```python
from build123d import *

# Parameters (mm, degrees)
SKETCH1_W             = 101.6
SKETCH1_H             = 25.4
BOSS_EXTRUDE1_DEPTH   = 9.525
SKETCH2_W             = 9.525
SKETCH2_H             = 3.175
SKETCH2_W_2           = 42.8625
SKETCH2_H_2           = 4.7625
CUT_EXTRUDE1_DEPTH    = 106.159144277
F_8_32_TAPPED_HOLE1_D = 3.4544


with BuildPart() as part:
    # Sketch1 → Boss-Extrude1 (new body)
    with BuildSketch(Plane.XY):
        with Locations((50.8, 12.7)):
            Rectangle(SKETCH1_W, SKETCH1_H)
    extrude(amount=BOSS_EXTRUDE1_DEPTH)

    # Sketch2 → Cut-Extrude1 (cut, through all)
    with BuildSketch(Plane(origin=(0, 25.4, 0), x_dir=(1, 0, 0), z_dir=(0, 1, 0))):
        with Locations((50.8, -7.9375)):
            Rectangle(SKETCH2_W, SKETCH2_H)
        with Locations((21.43125, -7.14375)):
            Rectangle(SKETCH2_W_2, SKETCH2_H_2)
        with Locations((80.16875, -7.14375)):
            Rectangle(SKETCH2_W_2, SKETCH2_H_2)
    extrude(amount=-CUT_EXTRUDE1_DEPTH, mode=Mode.SUBTRACT)

    # #8-32 Tapped Hole1 (through all)
    with Locations(Plane.XY.offset(6.35)):
        with Locations((50.8, 4.7625), (50.8, 20.6375)):
            Hole(F_8_32_TAPPED_HOLE1_D / 2)


solid = part.part
```
Input: part model. Units: mm. Frame: model coordinates. A direction names the side the tool comes from. Round coordinates to 2 decimals unless told otherwise and drop trailing zeros. Order: outer loops, then holes, each group sorted by start corner. A loop starts at its lowest first (then second) coordinate and runs counter-clockwise, first axis right, second up. Notation, with made-up numbers: (-2.75, 70) - (47.25, 70) arc R23 cw to (47.25, 98) - close; hole circle Ø10 at (18, 19.25). An arc over 180 degrees is marked (long way). One line per question, with ' | ' between items. Start each with the question number.
1) Set-up query: faces 4 (the flat face through (80, 13, 4.762)), 5 (the flat face through (50, 0, 3)), 6 (the flat face through (55.562, 13, 8)), 7 (the flat face through (21, 13, 4.762)). Return all of +Z, -Z, +X, -X, +Y, -Y with unobstructed straight access to the full face (end or side cutting, diameter ignored); none if empty.
2) Cut plane C-C, the plane x = 32. Return the cut outline in (y, z).
3) Cut plane A-A, the plane x = 50.8. Return the cut outline in (y, z), then the cut area to 3 significant figures.
4) Pull-direction query (X, two-part tool) for faces 1 (the flat face through (0, 13, 2)), 2 (the cylindrical face through (49.153, 5.281, 3.131)), 3 (the flat face through (50, 13, 0)); classes: +X half, -X half, draft (parallel to the pull), parting line (faces both ways), or undercut.
5) Ray query, probe 1 along Y at (x, z) = (50.8, 4.5); probe 2 along X at (y, z) = (11.25, 8.5); probe 3 along Y at (x, z) = (50.5, 2.75). Return the intervals inside material, ascending.
6) Contact query for flat-ended pins moving along their axis: P1, Ø2.5, axis at y = 16.5, z = 8, coming from the -X side; P2, Ø1.4, axis at y = 10, z = 7.5, coming from the +X side; P3, Ø2, axis at x = 50.8, y = 20.64, coming from the -Z side; P4, Ø5.5, axis at x = 50.8, y = 4.76, coming from the +Z side. Output: stop coordinate, or through.
Worked out:
1) face 4: +Z, +X, +Y, -Y | face 5: +Z, -Z, +X, -X, -Y | face 6: +Z, +Y, -Y | face 7: +Z, -X, +Y, -Y
2) outline: (0, 0) - (25.4, 0) - (25.4, 4.76) - (0, 4.76) - close
3) outline: (0, 0) - (3.04, 0) - (3.04, 6.35) - (0, 6.35) - close; (6.49, 0) - (18.91, 0) - (18.91, 6.35) - (6.49, 6.35) - close; (22.36, 0) - (25.4, 0) - (25.4, 6.35) - (22.36, 6.35) - close | area: 117 mm^2
4) face 1: -X half | face 2: undercut | face 3: draft
5) probe 1: y = 0 to 3.04, 6.49 to 18.91, 22.36 to 25.4 | probe 2: x = 42.86 to 46.04, 55.56 to 58.74 | probe 3: y = 0 to 3.06, 6.46 to 18.94, 22.34 to 25.4
6) P1: stops at x = 42.86 | P2: stops at x = 58.74 | P3: passes through | P4: stops at z = 6.35
